For this review, take the finished solid that the model builds, in its own axes (mm). Face numbers are marked on the shaded views. A direction names the side the tool comes from. Round coordinates to 2 decimals unless told otherwise and drop trailing zeros. Order: outer loops, then holes, each group sorted by start corner. A loop starts at its lowest first (then second) coordinate and runs counter-clockwise, first axis right, second up. Notation, with made-up numbers: (12, -38.5) -> (64, -38.5) arc R13 ccw to (64, -21.5) -> close; hole circle Ø7 at (-16.75, 62.5). An arc over 180 degrees is marked (long way). Answer in a Markdown table with one row per item.
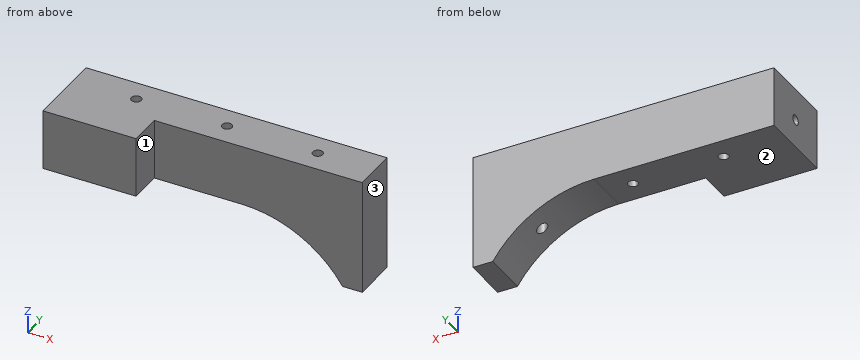
```python
from build123d import *

# Parameters (mm, degrees)
SKETCH1_R               = 1.65
BOSS_EXTRUDE1_DEPTH     = 38.1
SKETCH3_R               = 1.65
CUT_EXTRUDE1_DEPTH      = 20
CUT_EXTRUDE3_DEPTH      = 146.219699553
CUT_EXTRUDE3_DEPTH_BACK = 146.219699553


with BuildPart() as part:
    # Sketch1 → Boss-Extrude1 (new body)
    with BuildSketch(Plane.XY):
        Polygon((-7.90964601, 27), (-137.699495781, 27), (-137.699495781, 1), (-106.9, 1), (-106.9, 12), (-7.90964601, 12), align=None)
        with Locations((-116.9, 19.5)):
            Circle(SKETCH1_R, mode=Mode.SUBTRACT)
        with Locations((-86.9, 19.5)):
            Circle(SKETCH1_R, mode=Mode.SUBTRACT)
        with Locations((-56.9, 19.5)):
            Circle(SKETCH1_R, mode=Mode.SUBTRACT)
        with Locations((-26.9, 19.5)):
            Circle(SKETCH1_R, mode=Mode.SUBTRACT)
    extrude(amount=-BOSS_EXTRUDE1_DEPTH)

    # Sketch3 → Cut-Extrude1 (cut)
    with BuildSketch(Plane.ZY.offset(137.699495781)):
        with Locations((-10.698507709, 14)):
            Circle(SKETCH3_R)
    extrude(amount=-CUT_EXTRUDE1_DEPTH, mode=Mode.SUBTRACT)

    # Sketch4 → Cut-Extrude3 (cut, two sides: drawn at the far end of the back side and taken through both)
    with BuildSketch(Plane(origin=(0, 27, 0), x_dir=(1, 0, 0), z_dir=(0, 1, 0)).offset(-CUT_EXTRUDE3_DEPTH_BACK)):
        with BuildLine():
            ThreePointArc((-78.1, 20), (-59.07370241, 24.814775828), (-44.627772706, 38.1))
            Line((-44.627772706, 38.1), (-137.699495781, 38.1))
            Line((-137.699495781, 38.1), (-137.699495781, 20))
            Line((-137.699495781, 20), (-106.9, 20))
            Line((-106.9, 20), (-78.1, 20))
        make_face()
        Polygon((-38.1, 32.773477062), (-38.1, 28.046305235), (-38.1, 0), (-7.90964601, 0), (-7.90964601, 38.1), (-38.1, 38.1), align=None)
    extrude(amount=CUT_EXTRUDE3_DEPTH + CUT_EXTRUDE3_DEPTH_BACK, mode=Mode.SUBTRACT)


solid = part.part
```
Q1. Tool access review of the marked faces 1, 2 and 3: name each direction out of +Z, -Z, +X, -X, +Y, -Y from which nothing blocks a thin tool from reaching the whole face with its end or side.
Answer key:
| item | result |
|---|---|
| face 1 | +Z, -Z, +X, -Y |
| face 2 | -Z, -X, +Y, -Y |
| face 3 | +Z, -Z, +X, +Y, -Y |
Q2. Take a section at C-C, the plane y = 14. Write out the cut boundary in (x, z), then the cut area to 3 significant figures.
Answer key:
| item | result |
|---|---|
| outline | (-137.7, -20) -> (-78.1, -20) arc R40 cw to (-44.63, -38.1) -> (-38.1, -38.1) -> (-38.1, 0) -> (-137.7, 0) -> (-137.7, -9.05) -> (-117.7, -9.05) -> (-117.7, -12.35) -> (-137.7, -12.35) -> close |
| area | 2,220 mm^2 |
Q3. Take a section at D-D, the plane y = 19.5. Write out the cut boundary in (x, z), then the cut area to 3 significant figures.
Answer key:
| item | result |
|---|---|
| outline | (-137.7, -20) -> (-118.55, -20) -> (-118.55, 0) -> (-137.7, 0) -> close; (-115.25, -20) -> (-88.55, -20) -> (-88.55, 0) -> (-115.25, 0) -> close; (-85.25, -20) -> (-78.1, -20) arc R40 cw to (-58.55, -25.1) -> (-58.55, 0) -> (-85.25, 0) -> close; (-55.25, -27.17) arc R40 cw to (-44.63, -38.1) -> (-38.1, -38.1) -> (-38.1, 0) -> (-55.25, 0) -> close |
| area | 2,070 mm^2 |
Q4. To check wall thickness, follow probe 1 along Y at (x, z) = (-116.9, -8); probe 2 along Y at (x, z) = (-86.9, -6.25); probe 3 along Z at (x, y) = (-121.5, 24.5). State the ranges of each line that lie inside material, in increasing order.
Answer key:
| item | result |
|---|---|
| probe 1 | y = 1 to 17.85, 21.15 to 27 |
| probe 2 | y = 12 to 17.85, 21.15 to 27 |
| probe 3 | z = -20 to 0 |
Q5. Take a section at A-A, the plane z = -17. Write out the cut boundary in (x, y), then the cut area to 3 significant figures.
Answer key:
| item | result |
|---|---|
| outline | (-137.7, 1) -> (-106.9, 1) -> (-106.9, 12) -> (-38.1, 12) -> (-38.1, 27) -> (-137.7, 27) -> close; hole circle Ø3.3 at (-116.9, 19.5); hole circle Ø3.3 at (-86.9, 19.5); hole circle Ø3.3 at (-56.9, 19.5) |
| area | 1,810 mm^2 |
Q6. Take a section at B-B, the plane x = -86.9. Write out the cut boundary in (y, z).
Answer key:
| item | result |
|---|---|
| outline | (12, -20) -> (17.85, -20) -> (17.85, 0) -> (12, 0) -> close; (21.15, -20) -> (27, -20) -> (27, 0) -> (21.15, 0) -> close |
Q7. Clearance check with flat-ended pins moving along their axes: pin 1 Ø2 at (x, y) = (-86.9, 19.5) entering from +Z; pin 2 Ø3.5 at (y, z) = (5, -7) entering from +X; pin 3 Ø8 at (x, y) = (-102, 11) entering from -Z. State where each tip first meets the part, or that it passes through.
Answer key:
| item | result |
|---|---|
| pin 1 | passes through |
| pin 2 | stops at x = -106.9 |
| pin 3 | stops at z = -20 |
